For this review, take the finished solid that the model builds, in its own axes (mm). A direction names the side the tool comes from. Coordinates: 2 decimals unless noted, no trailing zeros. Order: outer loops, then holes, each group sorted by start corner. A loop starts at its lowest first (then second) coordinate and runs counter-clockwise, first axis right, second up. Notation, with made-up numbers: (36.25, 46) - (60.25, 46) arc R25 cw to (60.25, 82) - close; hole circle Ø10 at (-15.5, -14.5). An arc over 180 degrees is marked (long way). One line per item, written item: value. Start each with the question number.
(1) To check wall thickness, follow line 1 along X through (y, z) = (33.25, 1.5); line 2 along Y through (x, z) = (4, 1.6); line 3 along X through (y, z) = (26.5, 3.8). State the ranges of each line that lie inside material, in increasing order.
(2) Clearance check with flat-ended pins moving along their axes: pin 1 (3.5 mm diameter, centred on x = 3, y = 14, fed in from +Z); pin 2 (0.6 mm diameter, centred on y = 17, z = 3, fed in from -X). State where each tip first meets the part, or that it passes through.
(3) For faces 4 (the flat face through (14, 36, 2)), 5 (the flat face through (7, 18, 3)), list the 3-axis set-ups (+Z, -Z, +X, -X, +Y, -Y) from which the entire face can be reached by the end or side of a thin tool; tool diameter is ignored.
(4) Consider section C-C on x = 5.5. Write out the cut boundary in (y, z).
(5) Consider section B-B on y = 5.5. Write out the cut boundary in (x, z), then the cut area to 3 significant figures.
(6) Mouldability with a two-part tool opening along Y and no side actions: class faces 1 (the cylindrical face through (2.59, 0.87, 1.01)), 2 (the flat face through (14, 0, 2)), 3 (the flat face through (11, 18, 0)) as released by +Y, released by -Y, zero draft, split by the parting line, or undercut.
(7) Consider section A-A on y = 33.25. Write out the cut boundary in (x, z), then the cut area to 3 significant figures.
```python
from build123d import *

# Parameters (mm, degrees)
SKETCH_W       = 22
SKETCH_H       = 36
PAD_DEPTH      = 2
SKETCH001_R    = 1.925
HOLE_DEPTH     = 86.475848
PAD001_DEPTH   = 2
PAD001_FACE8_W = 32
PAD001_FACE8_H = 2
PAD002_DEPTH   = 10
PAD002_FACE9_W = 36
PAD002_FACE9_H = 2
PAD003_DEPTH   = 3


with BuildPart() as part:
    # Sketch → Pad (new body)
    with BuildSketch(Plane.XY):
        with Locations((11, 18)):
            Rectangle(SKETCH_W, SKETCH_H)
    extrude(amount=PAD_DEPTH)

    # Sketch001 (on Face6 of Pad) → Hole (cut, through all)
    with BuildSketch(Plane.XY.offset(2)):
        with Locations((3.010433, 2.75)):
            Circle(SKETCH001_R)
    hole = extrude(amount=-HOLE_DEPTH, mode=Mode.SUBTRACT)

    # Mirrored: Hole across Sketch001 Axis0
    add(hole.mirror(Plane(origin=(0, 18, 2), x_dir=(0, 0, 1), z_dir=(0, 1, 0))), mode=Mode.SUBTRACT)

    # Sketch002 (on Face5 of Mirrored) → Pad001 (join)
    with BuildSketch(Plane.XY.offset(2)):
        Polygon((10, 36), (10, 34), (20, 34), (20, 2), (10, 2), (10, 0), (22, 0), (22, 36), align=None)
    extrude(amount=PAD001_DEPTH)

    # Pad001 Face8 → Pad002 (add)
    with BuildSketch(Plane(origin=(20, 18, 3), x_dir=(0, 1, 0), z_dir=(-1, 0, 0))):
        Rectangle(PAD001_FACE8_W, PAD001_FACE8_H)
    extrude(amount=PAD002_DEPTH)

    # Pad002 Face9 → Pad003 (add)
    with BuildSketch(Plane(origin=(10, 18, 3), x_dir=(0, 1, 0), z_dir=(-1, 0, 0))):
        Rectangle(PAD002_FACE9_W, PAD002_FACE9_H)
    extrude(amount=PAD003_DEPTH)


solid = part.part
```
Geometry check:
1. line 1: x = 0 to 1.09, 4.94 to 22
1. line 2: y = 0 to 1.1, 4.4 to 31.6, 34.9 to 36
1. line 3: x = 7 to 22
2. pin 1: stops at z = 2
2. pin 2: stops at x = 7
3. face 4: +Z, -Z, +X, -X, +Y
3. face 5: +Z, -X, +Y, -Y
4. outline: (0, 0) - (36, 0) - (36, 2) - (0, 2) - close
5. outline: (0, 0) - (22, 0) - (22, 4) - (7, 4) - (7, 2) - (0, 2) - close
5. area: 74.0 mm^2
6. face 1: undercut
6. face 2: released by -Y
6. face 3: zero draft
7. outline: (0, 0) - (1.09, 0) - (1.09, 2) - (0, 2) - close; (4.94, 0) - (22, 0) - (22, 4) - (7, 4) - (7, 2) - (4.94, 2) - close
7. area: 66.3 mm^2
